```python
from build123d import *

# Parameters (mm, degrees)
F0_W     = 685.8
F0_H     = 254
F1_DEPTH = 254
F1_TAPER = -10
F2_W     = 772.1991061999
F2_H     = 340.3991061999
F3_DEPTH = 252.4125
F3_TAPER = 10


with BuildPart() as f1:
    # F0 (on Top) → F1 (new body)
    with BuildSketch(Plane.XY):
        with Locations((5.8371908963, -50.6961728707)):
            Rectangle(F0_W, F0_H)
    extrude(amount=F1_DEPTH, taper=F1_TAPER)

    # F2 (on face) → F3 (cut)
    with BuildSketch(Plane.XY.offset(254)):
        with Locations((5.8371908963, -50.6961728707)):
            Rectangle(F2_W, F2_H)
    extrude(amount=-F3_DEPTH, taper=F3_TAPER, mode=Mode.SUBTRACT)


solid = f1.part
```
The listing builds one solid part. Answer for the finished solid, in the listing's coordinates (mm). Round coordinates to 2 decimals unless told otherwise and drop trailing zeros. Write item = value, one per line.
1) For a pull along X with two mould halves and no side action, classify faces 1 (the flat face through (0, -49, 1.588)), 2 (the flat face through (0, -49, 0)) as released by +X, released by -X, zero draft, split by the parting line, or undercut.
Check values:
face_1 = undercut
face_2 = zero draft
2) Given pin 1 (5 mm diameter, centred on y = 26.5, z = 215, fed in from -X); pin 2 (8 mm diameter, centred on y = 39, z = 111, fed in from -X); pin 3 (12 mm diameter, centred on y = 65.5, z = 151.5, fed in from -X), each flat-ended and moving along its own axis, determine where each tip first touches the part or whether it passes through.
Check values:
pin_1 = -375.41
pin_2 = -357.34
pin_3 = -364.83
3) Straight lines are drawn through the part: line 1 along Z through (x, y) = (238, -149); line 2 along X through (y, z) = (18.5, 134) (1 decimal); line 3 along X through (y, z) = (-47, 109.5) (1 decimal). For each, find the intervals that lie inside material, in ascending order. Write a range as [from, to].
Check values:
line_1 = [0, 1.59]
line_2 = [-360.7, -359.1], [370.8, 372.4]
line_3 = [-356.4, -354.8], [366.5, 368]
